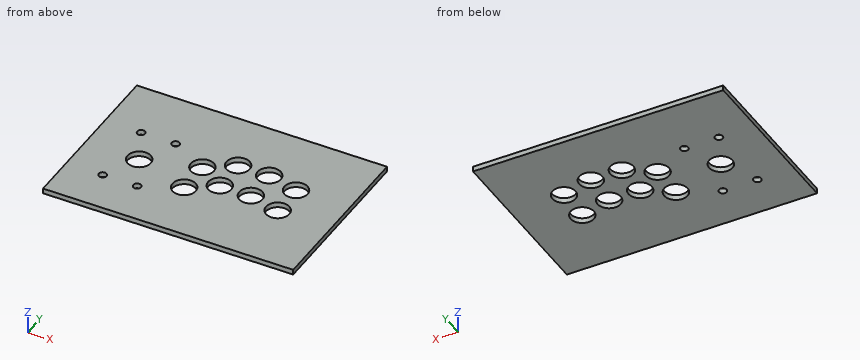
Autodesk Fusion 360 part; units mm, degrees
sketch "Sketch1" plane through (0, 0, 84.1556) normal (0, 0, 1) x (-1, 0, 0)
  circle A0 centre (86.7847, -20.259) radius 4.5
  circle A1 centre (-26.7153, -100.259) radius 13.5
  circle A2 centre (-98.7153, -52.259) radius 13.5
  circle A3 centre (-26.7153, -61.259) radius 13.5
  circle A4 centre (-62.7153, -100.259) radius 13.5
  circle A5 centre (46.7847, -20.259) radius 4.5
  circle A6 centre (46.7847, -102.259) radius 4.5
  circle A7 centre (3.7847, -80.259) radius 13.5
  circle A8 centre (-62.7153, -61.259) radius 13.5
  circle A9 centre (3.7847, -41.259) radius 13.5
  circle A10 centre (-98.7153, -91.259) radius 13.5
  circle A11 centre (66.7847, -61.259) radius 13.5
  circle A12 centre (86.7847, -102.259) radius 4.5
  line L0 (129.0347, 29.241) -> (-160.9653, 29.241)
  line L1 (-160.9653, 29.241) -> (-160.9653, -170.759)
  line L2 (-160.9653, -170.759) -> (129.0347, -170.759)
  line L3 (129.0347, -170.759) -> (129.0347, 29.241)
  circle A13 centre (66.7847, -61.259) radius 13.5
  circle A14 centre (86.7847, -102.259) radius 4.5
  circle A15 centre (46.7847, -102.259) radius 4.5
  circle A16 centre (86.7847, -20.259) radius 4.5
  circle A17 centre (46.7847, -20.259) radius 4.5
  circle A18 centre (3.7847, -41.259) radius 13.5
  circle A19 centre (3.7847, -80.259) radius 13.5
  circle A20 centre (-26.7153, -61.259) radius 13.5
  circle A21 centre (-26.7153, -100.259) radius 13.5
  circle A22 centre (-62.7153, -100.259) radius 13.5
  circle A23 centre (-62.7153, -61.259) radius 13.5
  circle A24 centre (-98.7153, -52.259) radius 13.5
  circle A25 centre (-98.7153, -91.259) radius 13.5
extrude "Extrude1" add sketch "Sketch1" along normal blind 6
equation "d148 = mat_thickness_6"
equation "mat_thickness_6 = 6 mm"
Part model, mm, in its own coordinate system. Round coordinates to 2 decimals unless told otherwise and drop trailing zeros. Order: outer loops, then holes, each group sorted by start corner. A loop starts at its lowest first (then second) coordinate and runs counter-clockwise, first axis right, second up. Notation, with made-up numbers: (-29.5, 12.5) -> (11.5, 12.5) arc R23 ccw to (11.5, 43.5) -> close; hole circle Ø1 at (-24.5, 37). An arc over 180 degrees is marked (long way). Put each result on its own line as item: value.
Q1. Band-saw the part on C-C (x = 91). Give the cut face in (y, z).
From the geometry:
outline: (-29.24, 84.16) -> (41.18, 84.16) -> (41.18, 90.16) -> (-29.24, 90.16) -> close; (63.34, 84.16) -> (80.18, 84.16) -> (80.18, 90.16) -> (63.34, 90.16) -> close; (102.34, 84.16) -> (170.76, 84.16) -> (170.76, 90.16) -> (102.34, 90.16) -> close
Q2. Pin check, flat tip, straight feed: pin 1 Ø14.5 at (x, y) = (-86.78, 20.26) entering from +Z. Stop position of the tip, or through.
From the geometry:
pin 1: stops at z = 90.16
Q3. Band-saw the part on B-B (z = 88.7). State how many separate pieces and enclosed holes the cut face has, and give its area (3 significant figures).
From the geometry:
separate pieces: 1
enclosed holes: 13
area: 52,600 mm2
Q4. Band-saw the part on A-A (x = 1). Give the cut face in (y, z), and give its area (3 significant figures).
From the geometry:
outline: (-29.24, 84.16) -> (28.64, 84.16) -> (28.64, 90.16) -> (-29.24, 90.16) -> close; (53.88, 84.16) -> (67.64, 84.16) -> (67.64, 90.16) -> (53.88, 90.16) -> close; (92.88, 84.16) -> (170.76, 84.16) -> (170.76, 90.16) -> (92.88, 90.16) -> close
area: 897 mm2
Q5. Wall check: line 1 (Y direction, x = 64, z = 89.35); line 2 (Y direction, x = 72.5, z = 87.35); line 3 (X direction, y = 43, z = 85.15). Give the ranges that are in metal, low to high. Write a range as [from, to].
From the geometry:
line 1: y = [-29.24, 47.82], [74.7, 86.82], [113.7, 170.76]
line 2: y = [-29.24, 51.96], [70.56, 90.96], [109.56, 170.76]
line 3: x = [-129.03, -17.17], [9.6, 88.89], [108.54, 160.97]
